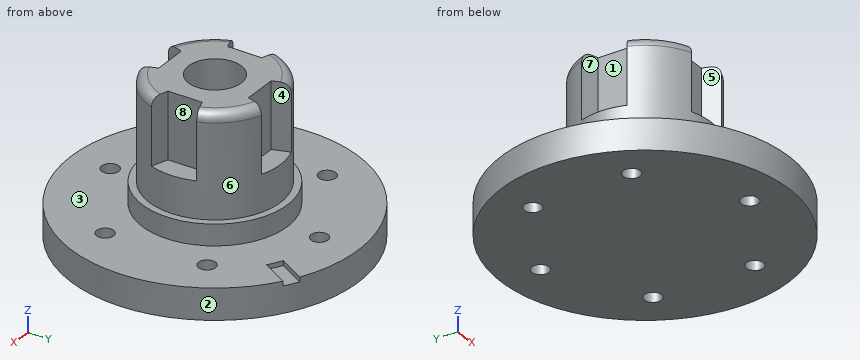
from build123d import *

# Parameters (mm, degrees)
SKETCH_1_R          = 18.5
SKETCH_1_R_2        = 1.1
EXTRUDE_1_DEPTH     = 4
SKETCH_3_R          = 8.45
EXTRUDE_3_DEPTH     = 15.9
FILLET_1_R          = 1.2
CUT_EXTRUDE_1_DEPTH = 8.5
SKETCH_5_R          = 9.35
EXTRUDE_4_DEPTH     = 2.7
SKETCH_6_R          = 1.1
CUT_EXTRUDE_2_DEPTH = 33.871111998
SKETCH_7_R          = 3.4
CUT_EXTRUDE_3_DEPTH = 6.5
CUT_EXTRUDE_START   = 4
CUT_EXTRUDE_5_DEPTH = 0.6


with BuildPart() as part:
    # Эскиз1 → Бобышка-Вытянуть1 (new body)
    with BuildSketch(Plane.XY):
        Circle(SKETCH_1_R)
        with Locations((0, 13.5)):
            Circle(SKETCH_1_R_2, mode=Mode.SUBTRACT)
        with Locations((-11.985507699, -6.212697095)):
            Circle(SKETCH_1_R_2, mode=Mode.SUBTRACT)
        with Locations((11.985507699, -6.212697095)):
            Circle(SKETCH_1_R_2, mode=Mode.SUBTRACT)
    extrude(amount=EXTRUDE_1_DEPTH)

    # Эскиз3 → Бобышка-Вытянуть3 (add)
    with BuildSketch(Plane.XY.offset(4)):
        Circle(SKETCH_3_R)
    extrude(amount=EXTRUDE_3_DEPTH)

    # Скругление1
    fillet_1_edges = [part.edges().sort_by_distance(p)[0] for p in [
        (-8.45, 0, 19.9),
    ]]
    fillet(fillet_1_edges, radius=FILLET_1_R)

    # Эскиз4 → Вырез-Вытянуть1 (cut)
    with BuildSketch(Plane.XY.offset(19.9)):
        with BuildLine():
            Line((-2.2, 5.799999981), (-2.931860794, 7.978357743))
            ThreePointArc((-2.931860794, 7.978357743), (-6.37e-07, 8.5), (2.931859599, 7.978358183))
            Line((2.931859599, 7.978358183), (2.2, 5.800000019))
            Line((2.2, 5.800000019), (-2.2, 5.799999981))
        make_face()
        with BuildLine():
            Line((5.799999981, 2.2), (7.978357743, 2.931860794))
            ThreePointArc((7.978357743, 2.931860794), (8.5, 6.37e-07), (7.978358183, -2.931859599))
            Line((7.978358183, -2.931859599), (5.800000019, -2.2))
            Line((5.800000019, -2.2), (5.799999981, 2.2))
        make_face()
        with BuildLine():
            Line((2.2, -5.799999981), (2.931860794, -7.978357743))
            ThreePointArc((2.931860794, -7.978357743), (6.37e-07, -8.5), (-2.931859599, -7.978358183))
            Line((-2.931859599, -7.978358183), (-2.2, -5.800000019))
            Line((-2.2, -5.800000019), (2.2, -5.799999981))
        make_face()
        with BuildLine():
            Line((-5.799999981, -2.2), (-7.978357743, -2.931860794))
            ThreePointArc((-7.978357743, -2.931860794), (-8.5, -6.37e-07), (-7.978358183, 2.931859599))
            Line((-7.978358183, 2.931859599), (-5.800000019, 2.2))
            Line((-5.800000019, 2.2), (-5.799999981, -2.2))
        make_face()
    extrude(amount=-CUT_EXTRUDE_1_DEPTH, mode=Mode.SUBTRACT)

    # Эскиз5 → Бобышка-Вытянуть4 (add)
    with BuildSketch(Plane.XY.offset(4)):
        with Locations(Location((0, 0, 0), (0, 0, 180))):
            Circle(SKETCH_5_R)
    extrude(amount=EXTRUDE_4_DEPTH)

    # Эскиз6 → Вырез-Вытянуть2 (cut, through all)
    with BuildSketch(Plane(origin=(0, 0, 0), x_dir=(-1, 0, 0), z_dir=(0, 0, -1))):
        with Locations((-11.691342951, 6.75)):
            Circle(SKETCH_6_R)
        with Locations((11.691342951, 6.75)):
            Circle(SKETCH_6_R)
        with Locations((0, -13.5)):
            Circle(SKETCH_6_R)
    extrude(amount=-CUT_EXTRUDE_2_DEPTH, mode=Mode.SUBTRACT)

    # Эскиз7 → Вырез-Вытянуть3 (cut)
    with BuildSketch(Plane.XY.offset(19.9)):
        Circle(SKETCH_7_R)
    extrude(amount=-CUT_EXTRUDE_3_DEPTH, mode=Mode.SUBTRACT)

    # Эскиз8 → Вырез-Вытянуть5 (cut)
    with BuildSketch(Plane.XY.offset(CUT_EXTRUDE_START)):
        Polygon((8.116025404, 12.057368355), (10.116025404, 15.52146997), (8.383974596, 16.52146997), (6.383974596, 13.057368355), align=None)
    extrude(amount=-CUT_EXTRUDE_5_DEPTH, mode=Mode.SUBTRACT)


solid = part.part
Can you work these out from the model? Positions are in its coordinate system, mm. Face numbers are marked on the shaded views. A direction names the side the tool comes from. Coordinates: 2 decimals unless noted, no trailing zeros. Write each loop counter-clockwise with the first axis right and the second up, starting at its lowest first coordinate (ties: lowest second). Pieces come first, ordered by that corner, then holes.
Q1. Imagine slicing it at D-D, the plane y = 0. List the corners of the cut face in (x, z) for me, plus the area to 3 significant figures.
Results found:
outline: (-18.5, 0) - (18.5, 0) - (18.5, 4) - (9.35, 4) - (9.35, 6.7) - (8.45, 6.7) - (8.45, 11.4) - (5.8, 11.4) - (5.8, 19.9) - (3.4, 19.9) - (3.4, 13.4) - (-3.4, 13.4) - (-3.4, 19.9) - (-5.8, 19.9) - (-5.8, 11.4) - (-8.45, 11.4) - (-8.45, 6.7) - (-9.35, 6.7) - (-9.35, 4) - (-18.5, 4) - close
area: 332 mm2
Q2. Please list where these lines run through material, in increasing order: L1, parallel to Y at x = 0, z = 1.8; L2, parallel to Z at x = 2.5, y = 0.5; L3, parallel to Z at x = -2, y = 14.
Results found:
L1: y = -18.5 to -14.6, -12.4 to 12.4, 14.6 to 18.5
L2: z = 0 to 13.4
L3: z = 0 to 4
Q3. Imagine slicing it at A-A, the plane z = 15. List the corners of the cut face in (x, y) for me, plus the area to 3 significant figures.
Results found:
outline: (-7.93, -2.92) arc R8.45 ccw to (-2.92, -7.93) - (-2.2, -5.8) - (2.2, -5.8) - (2.92, -7.93) arc R8.45 ccw to (7.93, -2.92) - (5.8, -2.2) - (5.8, 2.2) - (7.93, 2.92) arc R8.45 ccw to (2.92, 7.93) - (2.2, 5.8) - (-2.2, 5.8) - (-2.92, 7.93) arc R8.45 ccw to (-7.93, 2.92) - (-5.8, 2.2) - (-5.8, -2.2) - close; hole circle Ø6.8 at (0, 0)
area: 136 mm2
Q4. Imagine slicing it at B-B, the plane x = 0. List the corners of the cut face in (y, z) for me.
Results found:
outline: (-18.5, 0) - (-14.6, 0) - (-14.6, 4) - (-18.5, 4) - close; (-12.4, 0) - (12.4, 0) - (12.4, 4) - (9.35, 4) - (9.35, 6.7) - (8.45, 6.7) - (8.45, 11.4) - (5.8, 11.4) - (5.8, 19.9) - (3.4, 19.9) - (3.4, 13.4) - (-3.4, 13.4) - (-3.4, 19.9) - (-5.8, 19.9) - (-5.8, 11.4) - (-8.45, 11.4) - (-8.45, 6.7) - (-9.35, 6.7) - (-9.35, 4) - (-12.4, 4) - close; (14.6, 0) - (18.5, 0) - (18.5, 4) - (14.6, 4) - close
Q5. Which directions (+Z, -Z, +X, -X, +Y, -Y) give clear straight access to the entire face, cutting with the end or side of a thin tool? Please do the marked faces 4, 5, 6, 7 and 8.
Results found:
face 4: +Z, +Y
face 5: +Z, -Y
face 6: +Z
face 7: +Z, -X
face 8: +Z, +X
Q6. For P1, Ø3, axis at x = 11.69, y = 6.75, coming from the +Z side; P2, Ø4, axis at x = 9.5, z = 16, coming from the +Y side; P3, Ø10, axis at y = -12.5, z = 4.5, coming from the -X side, each with a flat end and sliding along its axis, tell me the tip position at first contact or that it passes through.
Results found:
P1: stops at z = 4
P2: stops at y = 3.89
P3: stops at x = -16.9
Q7. If we mould it in two halves opening along Y, with no side actions, what happens to the marked faces 1, 2 and 3? For each: +Y half, -Y half, draft (parallel to the pull), parting line (faces both ways), or undercut.
Results found:
face 1: undercut
face 2: parting line
face 3: draft
Q8. Imagine slicing it at C-C, the plane y = -13.5. List the corners of the cut face in (x, z) for me.
Results found:
outline: (-12.65, 0) - (-1.1, 0) - (-1.1, 4) - (-12.65, 4) - close; (1.1, 0) - (12.65, 0) - (12.65, 4) - (1.1, 4) - close
